Source: CAD feature listing. Evaluate the final solid. Frame: model axes, mm. A direction names the side the tool comes from. Round coordinates to 2 decimals unless told otherwise and drop trailing zeros. Order: outer loops, then holes, each group sorted by start corner. A loop starts at its lowest first (then second) coordinate and runs counter-clockwise, first axis right, second up. Notation, with made-up numbers: (45, -11.5) -> (88, -11.5) arc R16 ccw to (88, 6.5) -> close; hole circle Ø4 at (-7.75, 53.25). An arc over 180 degrees is marked (long way). One line per item, written item: value. Start each with the question number.
1) Section B-B (x = -352.5). Return the cut outline in (y, z), and give its area (3 significant figures).
2) Section A-A (z = 33.5). Return the cut outline in (x, y).
3) Reachability of faces 1 (the face through (7, 0, 34)), 2 (the face through (7, -2, 33)) from +Z, -Z, +X, -X, +Y, -Y: full face, straight path, thin tool, end or side. Return the list, or none.
4) Ray query, L1, parallel to Y at x = -304, z = 50; L2, parallel to Z at x = -147.5, y = 0.5. Return the intervals inside material, ascending.
5) Section C-C (y = 15). Return the cut outline in (x, z).
6) Pin query (flat end, axial travel): P1, Ø14.5, axis at x = 66, y = 17, coming from the +Z side; P2, Ø0.6, axis at x = 214, y = -0.5, coming from the -Z side; P3, Ø1, axis at x = 426.5, y = -1, coming from the -Z side. Return the tip coordinate at first contact, or that it passes through.
```python
from build123d import *

# Parameters (mm, degrees)
BASE_FLANGE1_DEPTH = 500
FILLET1_R          = 5
SKETCH2_W          = 7
SKETCH2_H          = 35
CUT_EXTRUDE1_DEPTH = 10


# Sheet-metal steps are written as plain solids
with BuildPart() as part:
    # Sketch1 → Base-Flange1 (new, symmetric)
    with BuildSketch(Plane(origin=(0, 0, 0), x_dir=(0, 0, -1), z_dir=(1, 0, 0))):
        with BuildLine():
            Line((-65, 0), (-1.3, 0))
            ThreePointArc((-1.3, 0), (-0.380761184, 0.380761184), (0, 1.3))
            Line((0, 1.3), (0, 30))
            Line((0, 30), (2, 30))
            Line((2, 30), (2, 1.3))
            ThreePointArc((2, 1.3), (1.033452378, -1.033452378), (-1.3, -2))
            Line((-1.3, -2), (-65, -2))
            Line((-65, -2), (-65, 0))
        make_face()
    extrude(amount=BASE_FLANGE1_DEPTH, both=True)

    # Fillet1
    fillet1_edges = [part.edges().sort_by_distance(p)[0] for p in [
        (500, -1, 65),
        (-500, -1, 65),
        (500, 30, -1),
        (-500, 30, -1),
    ]]
    fillet(fillet1_edges, radius=FILLET1_R)

    # Sketch2 → Cut-Extrude1 (cut)
    with BuildSketch(Plane(origin=(0, 0, 0), x_dir=(1, 0, 0), z_dir=(0, 1, 0))):
        with Locations((-425, -36)):
            Rectangle(SKETCH2_W, SKETCH2_H)
        with Locations((-212.5, -36)):
            Rectangle(SKETCH2_W, SKETCH2_H)
        with Locations((0, -36)):
            Rectangle(SKETCH2_W, SKETCH2_H)
        with Locations((212.5, -36)):
            Rectangle(SKETCH2_W, SKETCH2_H)
        with Locations((425, -36)):
            Rectangle(SKETCH2_W, SKETCH2_H)
    extrude(amount=-CUT_EXTRUDE1_DEPTH, mode=Mode.SUBTRACT)


solid = part.part
```
Findings:
1. outline: (-2, 1.3) arc R3.3 ccw to (1.3, -2) -> (30, -2) -> (30, 0) -> (1.3, 0) arc R1.3 cw to (0, 1.3) -> (0, 65) -> (-2, 65) -> close
1. area: 192 mm2
2. outline: (-500, -2) -> (-428.5, -2) -> (-428.5, 0) -> (-500, 0) -> close; (-421.5, -2) -> (-216, -2) -> (-216, 0) -> (-421.5, 0) -> close; (-209, -2) -> (-3.5, -2) -> (-3.5, 0) -> (-209, 0) -> close; (3.5, -2) -> (209, -2) -> (209, 0) -> (3.5, 0) -> close; (216, -2) -> (421.5, -2) -> (421.5, 0) -> (216, 0) -> close; (428.5, -2) -> (500, -2) -> (500, 0) -> (428.5, 0) -> close
3. face 1: +Z, +X, -X, +Y
3. face 2: +Z, -Z, +X, -X, -Y
4. L1: -2 to 0
4. L2: -1.9 to 0.28
5. outline: (-500, -2) -> (500, -2) -> (500, 0) -> (-500, 0) -> close
6. P1: z = 0
6. P2: z = -1.64
6. P3: z = -1.47
